Can you work these out from the model? Positions are in its coordinate system, mm. A direction names the side the tool comes from. Coordinates: 2 decimals unless noted, no trailing zeros. Order: outer loops, then holes, each group sorted by start corner. A loop starts at its lowest first (then second) coordinate and runs counter-clockwise, first axis right, second up. Notation, with made-up numbers: (41, 42.25) -> (91, 42.25) arc R19 ccw to (91, 57.25) -> close; hole circle Ø1 at (-29, -3). An arc over 180 degrees is marked (long way). Answer as a JSON object with one key per item and string values. Group by question number.
(1) Which directions (+Z, -Z, +X, -X, +Y, -Y) give clear straight access to the entire face, cutting with the end or side of a thin tool? Please do faces 1 (the cylindrical face through (-4.573, 6.19, 3.705)), 2 (the cylindrical face through (2.513, 6.19, -5.322)), 3 (the cylindrical face through (0.9, 4.2, -2.86)), 4 (the flat face through (-3, 2, -6)), 5 (the cylindrical face through (-5.748, 6.19, -1.265)).
(2) I need wall thicknesses on line 1 (Z direction, x = 1, y = 2.5); line 2 (X direction, y = 6.5, z = -2); line 3 (X direction, y = 4.25, z = 0). Which ranges of each line are inside material? Lowest first, please.
(3) For pin 1 (0.5 mm diameter, centred on x = -6.5, z = -2, fed in from +Y); pin 2 (4 mm diameter, centred on x = -3.5, y = 6, fed in from +Z); pin 3 (4.5 mm diameter, centred on x = -5, z = 5, fed in from +Y); pin 4 (1 mm diameter, centred on x = -5, y = 1.5, fed in from -Z), each with a flat end and sliding along its axis, tell me the tip position at first contact or that it passes through.
(4) I want a section at D-D, the plane y = 1. List the corners of the cut face in (x, z) for me.
(5) I want a section at C-C, the plane z = 0. List the corners of the cut face in (x, y) for me, plus the area to 3 significant figures.
(6) I want a section at B-B, the plane x = -4. List the corners of the cut face in (y, z) for me.
(7) I want a section at A-A, the plane y = 7.5. List the corners of the cut face in (x, z) for me, plus the area to 3 significant figures.
(8) If we mould it in two halves opening along Z, with no side actions, what happens to faces 6 (the cylindrical face through (0.045, 6.19, 5.885)), 7 (the flat face through (0, 8, 0)), 8 (the flat face through (-5, 2, 4))? For each: pulls with the +Z half, pulls with the -Z half, needs draft (parallel to the pull), parting line crosses it, or undercut.
from build123d import *

# Parameters (mm, degrees)
SKETCH1_R           = 7.25
BOSS_EXTRUDE1_DEPTH = 2
BOSS_EXTRUDE2_DEPTH = 8.5
INDICATOR_DEPTH     = 0.5
FILLET1_R           = 0.5
SKETCH4_R           = 3
CUT_EXTRUDE2_DEPTH  = 8
CHAMFER1_SIZE       = 0.5


with BuildPart() as part:
    # Sketch1 → Boss-Extrude1 (new body)
    with BuildSketch(Plane(origin=(0, 0, 0), x_dir=(1, 0, 0), z_dir=(0, 1, 0))):
        with Locations(Location((0, 0, 0), (0, 0, 270))):
            Circle(SKETCH1_R)
    extrude(amount=BOSS_EXTRUDE1_DEPTH)

    # Sketch2 → Boss-Extrude2 (add)
    with BuildSketch(Plane(origin=(0, 2, 0), x_dir=(1, 0, 0), z_dir=(0, 1, 0))):
        with BuildLine():
            ThreePointArc((0, 7.25), (2.553471118, 5.302337412), (5.668278248, 4.520301063))
            ThreePointArc((5.668278248, 4.520301063), (5.737597521, 1.309569193), (7.068227363, -1.613276771))
            ThreePointArc((7.068227363, -1.613276771), (4.601195965, -3.669331339), (3.145657109, -6.532024292))
            ThreePointArc((3.145657109, -6.532024292), (0, -5.885150532), (-3.145657109, -6.532024292))
            ThreePointArc((-3.145657109, -6.532024292), (-4.601195965, -3.669331339), (-7.068227363, -1.613276771))
            ThreePointArc((-7.068227363, -1.613276771), (-5.737597521, 1.309569193), (-5.668278248, 4.520301063))
            ThreePointArc((-5.668278248, 4.520301063), (-2.553471118, 5.302337412), (0, 7.25))
        make_face()
    extrude(amount=BOSS_EXTRUDE2_DEPTH)

    # Sketch3 → Indicator (cut)
    with BuildSketch(Plane(origin=(0, 10.5, 0), x_dir=(1, 0, 0), z_dir=(0, 1, 0))):
        with BuildLine():
            Line((0.5, 5.482775584), (0.5, 1.482775584))
            ThreePointArc((0.5, 1.482775584), (0, 0.982775584), (-0.5, 1.482775584))
            Line((-0.5, 1.482775584), (-0.5, 5.482775584))
            ThreePointArc((-0.5, 5.482775584), (0, 5.982775584), (0.5, 5.482775584))
        make_face()
    extrude(amount=-INDICATOR_DEPTH, mode=Mode.SUBTRACT)

    # Fillet1
    fillet1_edges = [part.edges().sort_by_distance(p)[0] for p in [
        (0.5, 10, -3.482775584),
        (0, 10, -0.982775584),
        (-0.5, 10, -3.482775584),
        (0, 10, -5.982775584),
    ]]
    fillet(fillet1_edges, radius=FILLET1_R - 0.0001)  # a hair under: the kernel refuses the full size

    # Sketch4 → Cut-Extrude2 (cut)
    with BuildSketch(Plane(origin=(0, 0, 0), x_dir=(-1, 0, 0), z_dir=(0, -1, 0))):
        with Locations(Location((0, 0, 0), (0, 0, 90))):
            Circle(SKETCH4_R)
    extrude(amount=-CUT_EXTRUDE2_DEPTH, mode=Mode.SUBTRACT)

    # Chamfer1
    chamfer1_edges = [part.edges().sort_by_distance(p)[0] for p in [
        (0, 0, 3),
    ]]
    chamfer(chamfer1_edges, length=CHAMFER1_SIZE)


solid = part.part
Computed values:
{
 "1": {"face 1": "+Z, -X, +Y", "face 2": "-Z, +X, +Y", "face 3": "-Y", "face 4": "-Z, -X, +Y", "face 5": "-X, +Y"},
 "2": {"line 1": "z = -6.29 to -2.83, 2.83 to 5.95", "line 2": "x = -5.61 to -2.24, 2.24 to 5.61", "line 3": "x = -6.16 to -3, 3 to 6.16"},
 "3": {"pin 1": "stops at y = 2", "pin 2": "stops at z = 6.53", "pin 3": "stops at y = 10.5", "pin 4": "stops at z = -5.68"},
 "4": {"outline": "circle Ø14.5 at (0, 0); hole circle Ø6 at (0, 0)"},
 "5": {"outline": "(-7.25, 0) -> (-3.5, 0) -> (-3, 0.5) -> (-3, 8) -> (3, 8) -> (3, 0.5) -> (3.5, 0) -> (7.25, 0) -> (7.25, 2) -> (6.16, 2) -> (6.16, 10.5) -> (-6.16, 10.5) -> (-6.16, 2) -> (-7.25, 2) -> close", "area": "85.4 mm2"},
 "6": {"outline": "(0, -6.05) -> (2, -6.05) -> (2, -4.77) -> (10.5, -4.77) -> (10.5, 4.53) -> (2, 4.53) -> (2, 6.05) -> (0, 6.05) -> close"},
 "7": {"outline": "(-7.07, 1.61) arc R7.97 cw to (-5.67, -4.52) arc R7.97 cw to (0, -7.25) arc R7.97 cw to (5.67, -4.52) arc R7.97 cw to (7.07, 1.61) arc R7.97 cw to (3.15, 6.53) arc R7.97 cw to (-3.15, 6.53) arc R7.97 cw to start; hole circle Ø6 at (0, 0)", "area": "96.4 mm2"},
 "8": {"face 6": "pulls with the +Z half", "face 7": "undercut", "face 8": "needs draft"}
}
